from build123d import *

# Parameters (mm, degrees)
SKETCH_1_R          = 40
EXTRUDE_1_DEPTH     = 40
SKETCH_3_R          = 30
CUT_EXTRUDE_2_DEPTH = 35
F_20_0MM_1_REACH    = 100.524
F_20_0MM_1_BORE_R   = 10


with BuildPart() as part:
    # 草圖1 → 填料-伸長1 (new body)
    with BuildSketch(Plane(origin=(0, 0, 0), x_dir=(1, 0, 0), z_dir=(0, 1, 0))):
        with Locations(Location((0, 0, 0), (0, 0, 270))):
            Circle(SKETCH_1_R)
    extrude(amount=EXTRUDE_1_DEPTH)

    # 草圖3 → 除料-伸長2 (cut)
    with BuildSketch(Plane(origin=(0, 40, 0), x_dir=(1, 0, 0), z_dir=(0, 1, 0))):
        with Locations(Location((0, 0, 0), (0, 0, 270))):
            Circle(SKETCH_3_R)
    extrude(amount=-CUT_EXTRUDE_2_DEPTH, mode=Mode.SUBTRACT)

    # Ø20.0mm 定位孔1 bore (on position points) → Ø20.0mm 定位孔1 (cut, up to next)
    with BuildSketch(Plane(origin=(-21.744758151, 21.94181737, 33.573285406), x_dir=(0.839332135156, 0, 0.543618953768), z_dir=(-0.543618953768, 0, 0.839332135156)), mode=Mode.PRIVATE) as f_20_0mm_1_sk1:
        Circle(F_20_0MM_1_BORE_R)
    f_20_0mm_1_tool1 = extrude(f_20_0mm_1_sk1.sketch, amount=-F_20_0MM_1_REACH, mode=Mode.PRIVATE) & part.part
    add(f_20_0mm_1_tool1.solids().sort_by_distance((-21.744758, 21.941817, 33.573285))[0], mode=Mode.SUBTRACT)


solid = part.part
Here's how the part is built. I have some questions about the finished solid (model axes, mm). A direction names the side the tool comes from. Round coordinates to 2 decimals unless told otherwise and drop trailing zeros. Order: outer loops, then holes, each group sorted by start corner. A loop starts at its lowest first (then second) coordinate and runs counter-clockwise, first axis right, second up. Notation, with made-up numbers: (89, -17.5) -> (93, -17.5) arc R19 cw to (93, 1.5) -> close; hole circle Ø2 at (19.25, -14.5). An arc over 180 degrees is marked (long way). Return JSON: item names as keys, results as strings.
Q1. If we section it at B-B on x = 0: List the corners of the cut face in (y, z) for me, plus the area to 3 significant figures.
Filled sheet:
{"outline": "(0, -40) -> (40, -40) -> (40, -30) -> (5, -30) -> (5, 30) -> (40, 30) -> (40, 40) -> (0, 40) -> close", "area": "1,100 mm^2"}
Q2. Which directions (+Z, -Z, +X, -X, +Y, -Y) give clear straight access to the entire face, cutting with the end or side of a thin tool? Please do faces 4 (the flat face through (30, 40, 6)), 5 (the cylindrical face through (1.32, 22.74, -29.97)).
Filled sheet:
{"face 4": "+Z, -Z, +X, -X, +Y", "face 5": "+Y"}
Q3. I need wall thicknesses on line 1 along X through (y, z) = (16, 0); line 2 along Y through (x, z) = (10.5, -21); line 3 along Z through (x, y) = (-12.5, 12). Which ranges of each line are inside material? Lowest first, please. Write a range as from..to.
Filled sheet:
{"line 1": "x = -40..-30, 30..40", "line 2": "y = 0..5", "line 3": "z = -38..-27.27, 27.27..38"}
Q4. If we mould it in two halves opening along Y, with no side actions, what happens to faces 1 (the flat face through (0, 5, 0)), 2 (the cylindrical face through (-10.852, 18.112, 33.747)), 3 (the flat face through (1, 0, -1))? For each: released by +Y, released by -Y, zero draft, split by the parting line, or undercut.
Filled sheet:
{"face 1": "released by +Y", "face 2": "undercut", "face 3": "released by -Y"}
Q5. If we section it at A-A on z = 0: List the corners of the cut face in (x, y) for me.
Filled sheet:
{"outline": "(-40, 0) -> (40, 0) -> (40, 40) -> (30, 40) -> (30, 5) -> (-30, 5) -> (-30, 40) -> (-40, 40) -> close"}
Q6. If we section it at D-D on x = -33: List the corners of the cut face in (y, z) for me.
Filled sheet:
{"outline": "(0, -22.61) -> (40, -22.61) -> (40, 22.61) -> (0, 22.61) -> close"}
Q7. For pin 1 Ø12 at (y, z) = (6, -15) entering from +X; pin 2 Ø10 at (x, y) = (-9, 6) entering from -Z; pin 3 Ø10 at (y, z) = (29, 1) entering from -X, each with a flat end and sliding along its axis, tell me the tip position at first contact or that it passes through.
Filled sheet:
{"pin 1": "stops at x = 38.97", "pin 2": "stops at z = -39.8", "pin 3": "stops at x = -40"}
Q8. If we section it at C-C on y = 29: List the corners of the cut face in (x, z) for me.
Filled sheet:
{"outline": "(-27.35, 29.19) arc R40 ccw (long way) to (-15.46, 36.89) -> (-9.9, 28.32) arc R30 cw (long way) to (-21.79, 20.62) -> close"}
